Could you check a few things on this model? Use its own coordinates, in mm. Face numbers are marked on the shaded views. A direction names the side the tool comes from. Give positions to 0.01 mm unless a question says otherwise; leave off trailing zeros. Loops run counter-clockwise (first coordinate to the right, second up) from the corner with the lowest first, then second, coordinate; pieces in that order, holes last. Notation, with made-up numbers: (26.5, 55.5) -> (41.5, 55.5) arc R22 cw to (41.5, 70.5) -> close; hole circle Ø8 at (-20.5, 11). An arc over 180 degrees is marked (long way). Write item = value, one per line. Start each with the question number.
1) I want a section at D-D (z = -490). List the corners of the cut face in (x, y) for me.
2) If we mould it in two halves opening along X, with no side actions, what happens to the marked faces 4, 5, 6 and 7? For each: +X half, -X half, draft (parallel to the pull), parting line (faces both ways), or undercut.
3) On a 3-axis mill with a long thin cutter (end or side, diameter ignored), from which of +Z, -Z, +X, -X, +Y, -Y can I reach the whole of each face in a straight line? I mean the marked faces 1, 2 and 3. Say none if no direction works.
4) I want a section at B-B (z = -469.5). List the corners of the cut face in (x, y) for me, and give its area (3 significant figures).
5) I need wall thicknesses on probe 1 along Y at (x, z) = (-597, -474.5); probe 2 along X at (y, z) = (-28.5, -472); probe 3 along Z at (x, y) = (-587, -36). Which ranges of each line are inside material? Lowest first, please. Write a range as from..to.
6) I want a section at A-A (y = -3). List the corners of the cut face in (x, z) for me (3 decimals), and give its area (3 significant figures).
7) I want a section at C-C (y = -17). List the corners of the cut face in (x, z) for me (3 decimals).
8) I'm going to push flat-ended pins straight in: pin 1 Ø1 at (y, z) = (-17.5, -483.5) entering from -X; pin 2 Ø6 at (y, z) = (-5, -488) entering from +X; pin 3 Ø3.5 at (x, z) = (-596.5, -471.5) entering from -Y; pin 4 Ø1.5 at (x, z) = (-592, -467.5) entering from -Y. Where does each tip first touch, or does it pass through?
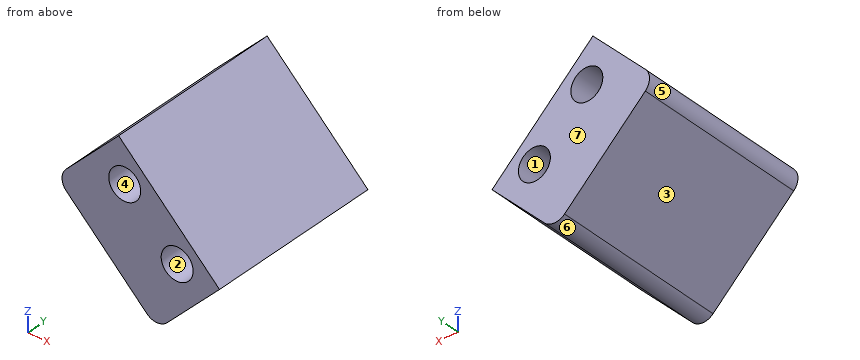
Autodesk Inventor part; units mm, degrees
ref_plane "YZ Plane" through (0, 0, 0) normal (1, 0, 0) x (0, 1, 0)
ref_plane "XZ Plane" through (0, 0, 0) normal (0, 1, 0) x (-1, 0, 0)
ref_plane "XY Plane" through (0, 0, 0) normal (0, 0, 1) x (1, 0, 0)
ref_plane "Work Plane1" through (49.1494, -37.6525, 49.2967) normal (0, 1, 0) x (-1, 0, 0)
sketch "Sketch2" plane through (49.1494, -37.6525, 49.2967) normal (0, 1, 0) x (-1, 0, 0)
  line L0 (662.4608, -525.6919) -> (646.2945, -509.5274)
  line L1 (143.1429, -6.4305) -> (69.9168, -79.6645)
  line L2 (623.8451, -531.9793) -> (639.991, -548.1234)
  line L3 (104.5272, -12.7179) -> (126.9766, 9.734)
  line L4 (646.2945, -509.5274) -> (662.4608, -525.6919)
  line L5 (662.4608, -525.6919) -> (639.991, -548.1234)
  line L6 (639.991, -548.1234) -> (623.8451, -531.9793)
  line L7 (623.8451, -531.9793) -> (646.2945, -509.5274)
  point P0 (49.1494, -49.2967)
  point P1 (69.9168, -79.6645)
extrude "Extrusion2" add sketch "Sketch2" along normal blind 40.64
sketch "Sketch3" plane through (49.1494, 2.9875, 49.2967) normal (0, 1, 0) x (1, 0, 0)
  circle A0 centre (-647.1931, 521.2017) radius 2.4765
  circle A1 centre (-635.5195, 532.8766) radius 2.4765
  point P0 (-49.1494, 49.2967)
hole "Hole1" at (-586.3701, 2.9875, -483.58) at (-598.0438, 2.9875, -471.905) direction (0, -1, 0) diameter 7.112 depth 10.414
sketch "Sketch4" plane through (49.1494, -37.6525, 49.2967) normal (0, -1, 0) x (1, 0, 0)
  circle A0 centre (-647.1931, -521.2017) radius 3.556
  circle A1 centre (-635.5195, -532.8766) radius 3.556
  point P0 (-49.1494, -49.2967)
extrude "Extrusion3" cut sketch "Sketch4" against normal blind 10.414
fillet "Fillet1" radius 3.175 2 edges at (-590.8417, -17.3325, -498.8268) (-613.3114, -17.3325, -476.3953)
sketch "Sketch5" plane through (-597.1451, -37.6525, -460.2307) normal (-0.7071, 0, 0.7071) x (0.7071, 0, 0.7071)
  line L0 (0, 40.64) -> (-19.6604, 40.64)
  line L1 (0, 0) -> (-3.175, 0)
  line L2 (-3.175, 0) -> (-3.175, 40.64)
  line L3 (-3.175, 40.64) -> (0, 40.64)
  line L4 (0, 40.64) -> (0, 0)
  point P0 (747.6829, 37.6525)
  dimension "d14" = 3.175
extrude "Extrusion4" cut sketch "Sketch5" against normal blind 46.0375
properties part number "Standoff"
Answer list:
q1.outline = (-599.68, -37.65) -> (-582.01, -37.65) -> (-582.01, 2.99) -> (-599.68, 2.99) -> close
q2.face_4 = undercut
q2.face_5 = -X half
q2.face_6 = parting line
q2.face_7 = draft
q3.face_1 = +Y
q3.face_2 = -Y
q3.face_3 = -Z, -X, +Y, -Y
q4.outline = (-606.42, -37.65) -> (-600.66, -37.65) -> (-600.66, -27.24) -> (-595.42, -27.24) -> (-595.42, -37.65) -> (-592.37, -37.65) -> (-592.37, 2.99) -> (-595.42, 2.99) -> (-595.42, -7.43) -> (-600.66, -7.43) -> (-600.66, 2.99) -> (-606.42, 2.99) -> close
q4.area = 462 mm^2
q5.probe_1 = -27.24..-7.43
q5.probe_2 = -608.92..-601.6, -594.49..-589.87
q5.probe_3 = -494.99..-487.08, -480.08..-474.87
q6.outline = (-611.064, -474.148) arc R3.175 ccw to (-611.062, -478.64) -> (-593.087, -496.586) arc R3.175 ccw to (-588.598, -496.584) -> (-576.94, -484.926) -> (-599.39, -462.476) -> close; hole circle Ø7.112 at (-598.044, -471.905); hole circle Ø7.112 at (-586.37, -483.58)
q6.area = 541 mm^2
q7.outline = (-611.064, -474.148) arc R3.175 ccw to (-611.062, -478.64) -> (-593.087, -496.586) arc R3.175 ccw to (-588.598, -496.584) -> (-576.94, -484.926) -> (-599.39, -462.476) -> close
q8.pin_1 = -606.7
q8.pin_2 = -577.01
q8.pin_3 = -27.24
q8.pin_4 = through
